Input: part model. Units: mm. Frame: model coordinates. Round coordinates to 2 decimals unless told otherwise and drop trailing zeros. Order: outer loops, then holes, each group sorted by start corner. A loop starts at its lowest first (then second) coordinate and runs counter-clockwise, first axis right, second up.
Item 1: Cut plane A-A on z = -15.5. Output: boundary loops of the cut face in (x, y), then the cut area to 3 significant figures.
Item 2: Cut plane C-C on x = -17.5. Output: boundary loops of the cut face in (y, z).
Item 3: Line query: L1, parallel to X at y = 2.25, z = 1; L2, parallel to X at y = -1.5, z = 16; L3, parallel to Z at x = -49, y = -1.9. Output: solid intervals per line, ascending.
Item 4: Cut plane B-B on y = 1.7. Give the number of separate pieces and of enclosed holes in the cut face, then the cut area to 3 significant figures.
Item 5: First-contact query: pin 1 (2.5 mm diameter, centred on y = -0.5, z = 16.5, fed in from +X); pin 2 (1.5 mm diameter, centred on y = 1, z = -11, fed in from -X); pin 3 (1.5 mm diameter, centred on x = -56, y = 1, fed in from +Z). Flat tips, straight axial feed; report the tip coordinate or a pass-through.
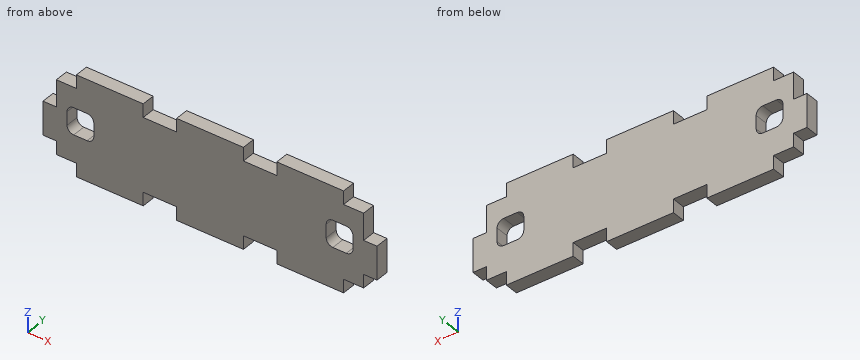
```python
from build123d import *

# Parameters (mm, degrees)
SKETCH1_W           = 127
SKETCH1_H           = 38.1
BOSS_EXTRUDE1_DEPTH = 2.54
SKETCH2_W           = 5.08
SKETCH2_H           = 10.16
SKETCH2_H_2         = 15.24
CUT_EXTRUDE1_DEPTH  = 5.08
SKETCH3_W           = 12.7
SKETCH3_H           = 5.08
CUT_EXTRUDE2_DEPTH  = 5.08
SKETCH4_W           = 12.7
SKETCH4_H           = 5.08
CUT_EXTRUDE4_DEPTH  = 5.08
LPATTERN1_COUNT     = 2
LPATTERN1_PITCH     = 38.1
SKETCH7_W           = 116.84
SKETCH7_H           = 5.08
CUT_EXTRUDE7_DEPTH  = 5.08
SKETCH8_W           = 25.4
SKETCH8_H           = 5.08
BOSS_EXTRUDE2_DEPTH = 5.08
CUT_EXTRUDE8_DEPTH  = 5.08


with BuildPart() as part:
    # Sketch1 → Boss-Extrude1 (new body, symmetric)
    with BuildSketch(Plane(origin=(0, 0, 0), x_dir=(1, 0, 0), z_dir=(0, 1, 0))):
        Rectangle(SKETCH1_W, SKETCH1_H)
    extrude(amount=BOSS_EXTRUDE1_DEPTH, both=True)

    # Sketch2 → Cut-Extrude1 (cut)
    with BuildSketch(Plane(origin=(0, 2.54, 0), x_dir=(1, 0, 0), z_dir=(0, 1, 0))):
        with Locations((-60.96, 13.97)):
            Rectangle(SKETCH2_W, SKETCH2_H)
        with Locations((-60.96, -11.43)):
            Rectangle(SKETCH2_W, SKETCH2_H_2)
    cut_extrude1 = extrude(amount=-CUT_EXTRUDE1_DEPTH, mode=Mode.SUBTRACT)

    # Mirror1: Cut-Extrude1 across plane
    add(cut_extrude1.mirror(Plane(origin=(0, 0, 0), x_dir=(0, 0, 1), z_dir=(1, 0, 0))), mode=Mode.SUBTRACT)

    # Sketch3 → Cut-Extrude2 (cut)
    with BuildSketch(Plane(origin=(0, 2.54, 0), x_dir=(1, 0, 0), z_dir=(0, 1, 0))):
        with Locations((-57.15, -16.51)):
            Rectangle(SKETCH3_W, SKETCH3_H)
    cut_extrude2 = extrude(amount=-CUT_EXTRUDE2_DEPTH, mode=Mode.SUBTRACT)

    # Mirror2: Cut-Extrude2 across plane
    add(cut_extrude2.mirror(Plane(origin=(0, 0, 0), x_dir=(0, 0, 1), z_dir=(1, 0, 0))), mode=Mode.SUBTRACT)

    # Sketch4 → Cut-Extrude4 (cut)
    with BuildSketch(Plane(origin=(0, 2.54, 0), x_dir=(1, 0, 0), z_dir=(0, 1, 0))):
        with Locations((-19.05, -16.51)):
            Rectangle(SKETCH4_W, SKETCH4_H)
    cut_extrude4 = extrude(amount=-CUT_EXTRUDE4_DEPTH, mode=Mode.SUBTRACT)

    # LPattern1: Cut-Extrude4 ×2
    with Locations(*[(i * LPATTERN1_PITCH, 0, 0) for i in range(1, LPATTERN1_COUNT)]):
        add(cut_extrude4, mode=Mode.SUBTRACT)

    # Sketch7 → Cut-Extrude7 (cut)
    with BuildSketch(Plane(origin=(0, 2.54, 0), x_dir=(1, 0, 0), z_dir=(0, 1, 0))):
        with Locations((0, 16.51)):
            Rectangle(SKETCH7_W, SKETCH7_H)
    extrude(amount=-CUT_EXTRUDE7_DEPTH, mode=Mode.SUBTRACT)

    # Sketch8 → Boss-Extrude2 (add)
    with BuildSketch(Plane(origin=(0, 2.54, 0), x_dir=(1, 0, 0), z_dir=(0, 1, 0))):
        with Locations((-38.1, 16.51)):
            Rectangle(SKETCH8_W, SKETCH8_H)
        with Locations((0, 16.51)):
            Rectangle(SKETCH8_W, SKETCH8_H)
        with Locations((38.1, 16.51)):
            Rectangle(SKETCH8_W, SKETCH8_H)
    extrude(amount=-BOSS_EXTRUDE2_DEPTH)

    # Sketch9 → Cut-Extrude8 (cut)
    with BuildSketch(Plane(origin=(0, 2.54, 0), x_dir=(1, 0, 0), z_dir=(0, 1, 0))):
        with BuildLine():
            Line((-51.807363259, 3.81), (-46.727363259, 3.81))
            ThreePointArc((-46.727363259, 3.81), (-44.931312035, 3.066051224), (-44.187363259, 1.27))
            Line((-44.187363259, 1.27), (-44.187363259, -3.81))
            ThreePointArc((-44.187363259, -3.81), (-44.931312035, -5.606051224), (-46.727363259, -6.35))
            Line((-46.727363259, -6.35), (-51.807363259, -6.35))
            ThreePointArc((-51.807363259, -6.35), (-53.603414483, -5.606051224), (-54.347363259, -3.81))
            Line((-54.347363259, -3.81), (-54.347363259, 1.27))
            ThreePointArc((-54.347363259, 1.27), (-53.603414483, 3.066051224), (-51.807363259, 3.81))
        make_face()
    cut_extrude8 = extrude(amount=-CUT_EXTRUDE8_DEPTH, mode=Mode.SUBTRACT)

    # Mirror3: Cut-Extrude8 across plane
    add(cut_extrude8.mirror(Plane(origin=(0, 0, 0), x_dir=(0, 0, 1), z_dir=(1, 0, 0))), mode=Mode.SUBTRACT)


solid = part.part
```
From the geometry:
1. outline: (-50.8, -2.54) - (-25.4, -2.54) - (-25.4, 2.54) - (-50.8, 2.54) - close; (-12.7, -2.54) - (12.7, -2.54) - (12.7, 2.54) - (-12.7, 2.54) - close; (25.4, -2.54) - (50.8, -2.54) - (50.8, 2.54) - (25.4, 2.54) - close
1. area: 387 mm2
2. outline: (-2.54, -13.97) - (2.54, -13.97) - (2.54, 13.97) - (-2.54, 13.97) - close
3. L1: x = -63.5 to -54.35, -44.19 to 44.19, 54.35 to 63.5
3. L2: x = -50.8 to -25.4, -12.7 to 12.7, 25.4 to 50.8
3. L3: z = -19.05 to -3.81, 6.35 to 19.05
4. separate pieces: 1
4. enclosed holes: 2
4. area: 3,970 mm2
5. pin 1: stops at x = 50.8
5. pin 2: stops at x = -58.42
5. pin 3: stops at z = 13.97
